Could you check a few things on this model? Use its own coordinates, in mm. Face numbers are marked on the shaded views. A direction names the side the tool comes from. Round coordinates to 2 decimals unless told otherwise and drop trailing zeros. Loops run counter-clockwise (first coordinate to the right, second up) from the corner with the lowest first, then second, coordinate; pieces in that order, holes last. Notation, with made-up numbers: M -25.75,59 L 33.25,59 A16 cw 33.25,63 Z; hole C 2.5,-7 d7. An arc over 180 degrees is marked long. One line per item, written item: value. Start each with the question number.
Q1. Thinking about a two-plate mould opening in Y: for the marked faces 4, 5 and 6, which applies, released by +Y, released by -Y, zero draft, split by the parting line, or undercut?
Q2. I'm going to push flat-ended pins straight in: pin 1 Ø4.5 at (x, z) = (5.08, 28.7) entering from +Y; pin 2 Ø6.5 at (x, y) = (9, 8.5) entering from +Z; pin 3 Ø4 at (x, z) = (21.5, 17) entering from -Y. Where does each tip first touch, or does it pass through?
Q3. Imagine slicing it at C-C (x = 17.5). Please give me the cut outline in (y, z).
Q4. Which directions (+Z, -Z, +X, -X, +Y, -Y) give clear straight access to the entire face, cutting with the end or side of a thin tool? Please do the marked faces 1, 2 and 3.
Q5. Please list where these lines run through material, in increasing order: line 1 along Z through (x, y) = (27.5, -37); line 2 along Y through (x, z) = (18, 31); line 3 along Z through (x, y) = (2, -2).
Q6. Imagine slicing it at D-D (z = 28.5). Please give me the cut outline in (x, y).
Q7. Imagine slicing it at A-A (x = 5.08). Please give me the cut outline in (y, z).
Q8. Imagine slicing it at B-B (y = -41). Please give me the cut outline in (x, z), then the cut area to 3 significant figures.
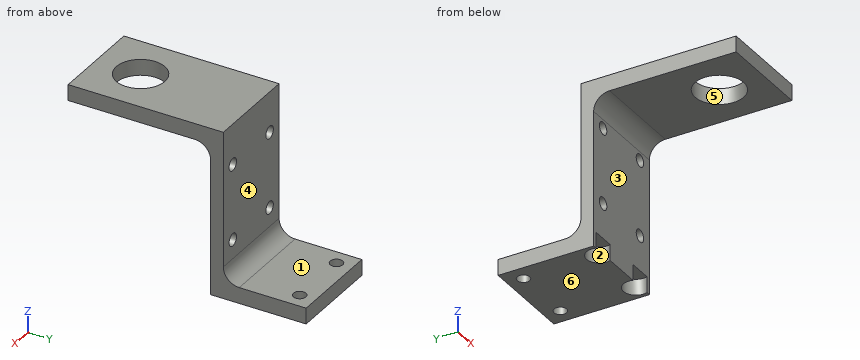
from build123d import *

# Parameters (mm, degrees)
BOSS_EXTRUDE1_DEPTH = 29.972
FILLET1_R           = 5.08
SKETCH3_R           = 2
SKETCH3_R_2         = 4
CUT_EXTRUDE1_DEPTH  = 5.08
SKETCH4_R           = 2
CUT_EXTRUDE2_DEPTH  = 29.972
SKETCH5_R           = 7.75
CUT_EXTRUDE3_DEPTH  = 5.08


with BuildPart() as part:
    # Sketch2 → Boss-Extrude1 (new body)
    with BuildSketch(Plane(origin=(0, 0, 0), x_dir=(0, 0, -1), z_dir=(1, 0, 0))):
        Polygon((6.609800113, 17.56515608), (6.609800113, -8.85084392), (-41.650199887, -8.85084392), (-41.650199887, -58.38084392), (-36.570199887, -58.38084392), (-36.570199887, -12.91484392), (11.689800113, -12.91484392), (11.689800113, 17.56515608), align=None)
    extrude(amount=BOSS_EXTRUDE1_DEPTH)

    # Fillet1
    fillet1_edges = [part.edges().sort_by_distance(p)[0] for p in [
        (14.986, -8.85084392, -6.609800113),
        (14.986, -12.91484392, 36.570199887),
    ]]
    fillet(fillet1_edges, radius=FILLET1_R)

    # Sketch3 → Cut-Extrude1 (cut)
    with BuildSketch(Plane(origin=(0, 0, -11.689800113), x_dir=(-1, 0, 0), z_dir=(0, 0, -1))):
        with Locations((-24.892, 12.48515608)):
            Circle(SKETCH3_R)
        with Locations((-5.08, 12.48515608)):
            Circle(SKETCH3_R)
        with Locations((-5.08, -11.64484392)):
            Circle(SKETCH3_R_2)
        with Locations((-24.892, -11.64484392)):
            Circle(SKETCH3_R_2)
    extrude(amount=-CUT_EXTRUDE1_DEPTH, mode=Mode.SUBTRACT)

    # Sketch4 → Cut-Extrude2 (cut)
    with BuildSketch(Plane.XZ.offset(12.91484392)):
        with Locations(Location((24.892, 4.566199887, 0), (0, 0, 270))):
            Circle(SKETCH4_R)
        with Locations(Location((5.08, 4.566199887, 0), (0, 0, 270))):
            Circle(SKETCH4_R)
        with Locations(Location((24.892, 28.696199887, 0), (0, 0, 270))):
            Circle(SKETCH4_R)
        with Locations(Location((5.08, 28.696199887, 0), (0, 0, 270))):
            Circle(SKETCH4_R)
    extrude(amount=-CUT_EXTRUDE2_DEPTH, mode=Mode.SUBTRACT)

    # Sketch5 → Cut-Extrude3 (cut)
    with BuildSketch(Plane(origin=(0, 0, 36.570199887), x_dir=(-1, 0, 0), z_dir=(0, 0, -1))):
        with Locations((-14.986, -44.15684392)):
            Circle(SKETCH5_R)
    extrude(amount=-CUT_EXTRUDE3_DEPTH, mode=Mode.SUBTRACT)


solid = part.part
Report:
1. face 4: released by +Y
1. face 5: undercut
1. face 6: zero draft
2. pin 1: stops at y = -8.85
2. pin 2: stops at z = -6.61
2. pin 3: stops at y = -12.91
3. outline: M -58.38,36.57 L -51.49,36.57 L -51.49,41.65 L -58.38,41.65 Z; M -36.83,36.57 L -17.99,36.57 A5.08 cw -12.91,31.49 L -12.91,-11.69 L 17.57,-11.69 L 17.57,-6.61 L -3.77,-6.61 A5.08 cw -8.85,-1.53 L -8.85,41.65 L -36.83,41.65 Z
4. face 1: +Z, +X, -X, +Y
4. face 2: -Z
4. face 3: -Z, +X, -X, -Y
5. line 1: z = 36.57 to 41.65
5. line 2: y = -12.91 to -8.85
5. line 3: z = -11.69 to -6.61
6. outline: M 0,-12.91 L 3.09,-12.91 L 3.09,-8.85 L 0,-8.85 Z; M 7.07,-12.91 L 22.9,-12.91 L 22.9,-8.85 L 7.07,-8.85 Z; M 26.88,-12.91 L 29.97,-12.91 L 29.97,-8.85 L 26.88,-8.85 Z
7. outline: M -58.38,36.57 L -17.99,36.57 A5.08 cw -12.91,31.49 L -12.91,30.7 L -8.85,30.7 L -8.85,41.65 L -58.38,41.65 Z; M -12.91,-6.61 L -7.64,-6.61 L -7.64,-11.69 L 10.49,-11.69 L 10.49,-6.61 L -3.77,-6.61 A5.08 cw -8.85,-1.53 L -8.85,2.57 L -12.91,2.57 Z; M -12.91,6.57 L -8.85,6.57 L -8.85,26.7 L -12.91,26.7 Z; M 14.49,-11.69 L 17.57,-11.69 L 17.57,-6.61 L 14.49,-6.61 Z
8. outline: M 0,36.57 L 7.91,36.57 L 7.91,41.65 L 0,41.65 Z; M 22.06,36.57 L 29.97,36.57 L 29.97,41.65 L 22.06,41.65 Z
8. area: 80.3 mm²
